```python
from build123d import *

# Parameters (mm, degrees)
F0_R     = 30
F1_DEPTH = 6.35
F3_D     = 10
F6_D     = 6.35
F7_D     = 4.5
F8_D     = 2.7051
F9_D     = 2.7051


with BuildPart() as f1:
    # F0 (on Top) → F1 (new body)
    with BuildSketch(Plane.XY):
        Polygon((-190, 60), (-130, 0), (130, 0), (190, 60), (190, 240), (130, 300), (-130, 300), (-190, 240), align=None)
        with Locations((0, 150)):
            Circle(F0_R, mode=Mode.SUBTRACT)
    extrude(amount=F1_DEPTH)

    # F3 (through all)
    with Locations(Plane.XY.offset(6.35)):
        with Locations((-125, 150), (125, 150)):
            Hole(F3_D / 2)

    # F6 (through all)
    with Locations(Plane.XY.offset(6.35)):
        with Locations((0, 218.14583), (59.016019942, 184.072915), (-59.016019942, 184.072915), (-59.016019942, 115.927085), (0, 81.85417), (59.016019942, 115.927085)):
            Hole(F6_D / 2)

    # F7 (through all)
    with Locations(Plane.XY.offset(6.35)):
        with Locations((-161.2489651369, 241.2489651369), (-131.2489651369, 271.2489651369), (-161.2489651369, 58.7510348631), (-131.2489651369, 28.7510348631), (131.2489651369, 28.7510348631), (161.2489651369, 58.7510348631), (161.2489651369, 241.2489651369), (131.2489651369, 271.2489651369)):
            Hole(F7_D / 2)

    # F8 (through all)
    with Locations(Plane.XY.offset(6.35)):
        with Locations((157.7549359697, 267.7549359697), (157.7549359697, 32.2450640303), (-157.7549359697, 32.2450640303), (-157.7549359697, 267.7549359697)):
            Hole(F8_D / 2)

    # F9 (through all)
    with Locations(Plane.XY.offset(6.35)):
        with Locations((-159.8994949366, 255.7573593129), (-145.7573593129, 269.8994949366), (-159.8994949366, 44.2426406871), (-145.7573593129, 30.1005050634), (145.7573593129, 30.1005050634), (159.8994949366, 44.2426406871), (145.7573593129, 269.8994949366), (159.8994949366, 255.7573593129)):
            Hole(F9_D / 2)


solid = f1.part
```
Design review of the part built by this model. Coordinates are the model's own, in mm. Coordinates: 2 decimals unless noted, no trailing zeros. Order: outer loops, then holes, each group sorted by start corner. A loop starts at its lowest first (then second) coordinate and runs counter-clockwise, first axis right, second up.
1) Take a section at A-A, the plane y = 150. Give the boundary of the cut face in (x, z), and give its area (4 significant figures).
2) Wall thickness on line 1 along Y through (x, z) = (-161.5, 4.25); line 2 along Y through (x, z) = (125, 4.75); line 3 along Y through (x, z) = (157, 1.75): over which ranges is each line inside the solid? List them lowest first.
3) Clearance check with a flat-ended pin moving along its axis: pin 1 (4 mm diameter, centred on x = -59.02, y = 184.07, fed in from +Z). State where the tip first meets the part, or that it passes through.
4) Mouldability with a two-part tool opening along X and no side actions: class faces 1 (the flat face through (-3, 119, 6.35)), 2 (the flat face through (-160, 30, 3)), 3 (the cylindrical face through (-6.503, 120.713, 3.131)), 4 (the cylindrical face through (120.381, 148.085, 3.131)) as +X half, -X half, draft (parallel to the pull), parting line (faces both ways), or undercut.
5) Take a section at B-B, the plane x = -125. Give the boundary of the cut face in (y, z), and give its area (3 significant figures).
6) Take a section at C-C, the plane z = 5. State how many separate pieces and enclosed holes the cut face has, and give its area (3 significant figures).
Returned:
1. outline: (-190, 0) - (-130, 0) - (-130, 6.35) - (-190, 6.35) - close; (-120, 0) - (-30, 0) - (-30, 6.35) - (-120, 6.35) - close; (30, 0) - (120, 0) - (120, 6.35) - (30, 6.35) - close; (130, 0) - (190, 0) - (190, 6.35) - (130, 6.35) - close
1. area: 1,905 mm2
2. line 1: y = 31.5 to 56.52, 60.99 to 239.01, 243.48 to 268.5
2. line 2: y = 0 to 145, 155 to 300
2. line 3: y = 27 to 31.12, 33.37 to 266.63, 268.88 to 273
3. pin 1: passes through
4. face 1: draft
4. face 2: -X half
4. face 3: undercut
4. face 4: undercut
5. outline: (0, 0) - (145, 0) - (145, 6.35) - (0, 6.35) - close; (155, 0) - (300, 0) - (300, 6.35) - (155, 6.35) - close
5. area: 1,840 mm2
6. separate pieces: 1
6. enclosed holes: 29
6. area: 103,000 mm2
